Can you work these out from the model? Positions are in its coordinate system, mm. A direction names the side the tool comes from. Round coordinates to 2 decimals unless told otherwise and drop trailing zeros. Loops run counter-clockwise (first coordinate to the right, second up) from the corner with the lowest first, then second, coordinate; pieces in that order, holes last.
Autodesk Inventor part; units mm, degrees
ref_plane "YZ Plane" through (0, 0, 0) normal (1, 0, 0) x (0, 1, 0)
ref_plane "XZ Plane" through (0, 0, 0) normal (0, 1, 0) x (-1, 0, 0)
ref_plane "XY Plane" through (0, 0, 0) normal (0, 0, 1) x (1, 0, 0)
sketch "Sketch1" plane through (0, 0, 0) normal (0, 1, 0) x (-1, 0, 0)
  line L0 (0, 0) -> (-20.3922, 0)
  line L1 (-20.3922, 0) -> (-20.3922, -40.9956)
  line L2 (-20.3922, -40.9956) -> (0, -40.9956)
  line L3 (0, -40.9956) -> (0, 0)
  line L4 (1.8083, 7.7679) -> (6.8846, 7.9604)
  line L5 (-22.5838, -48.6642) -> (-27.2554, -50.6597)
  line L6 (6.8846, 7.9604) -> (-27.2554, 7.9604)
  line L7 (-27.2554, 7.9604) -> (-27.2554, -50.6597)
  line L8 (-27.2554, -50.6597) -> (6.8846, -50.6597)
  line L9 (6.8846, -50.6597) -> (6.8846, 7.9604)
  circle A0 centre (-5.0927, 3.9878) radius 1.651
  circle A1 centre (-15.2781, 3.9878) radius 1.651
  circle A2 centre (-5.0927, -44.9834) radius 1.651
  circle A3 centre (-15.2781, -44.9834) radius 1.651
  dimension "d0" = 40.9956
  dimension "d2" = 7.9756
  dimension "d3" = 5.08
  dimension "d4" = 7.9756
  dimension "d5" = 5.08
  dimension "d6" = 3.302
  dimension "d7" = 3.302
  dimension "d8" = 3.302
  dimension "d9" = 3.302
  dimension "d24" = 6.8846
  dimension "d25" = 6.8633
extrude "Extrusion1" add sketch "Sketch1" along normal blind 7.62
sketch "Sketch2" plane through (0, 0, 0) normal (0, -1, 0) x (1, 0, 0)
  line L0 (27.2554, 7.9604) -> (27.2554, -50.6597)
  line L1 (27.2554, -42.6841) -> (-6.8846, -42.6841)
  line L2 (-6.8846, -42.6841) -> (-6.8846, -50.6597)
  line L3 (-6.8846, -50.6597) -> (27.2554, -50.6597)
  line L4 (27.2554, -50.6597) -> (27.2554, -42.6841)
  point P0 (0, 0)
extrude "Extrusion2" add sketch "Sketch2" along normal blind 38.862
sketch "Sketch3" plane through (27.2554, 0, 7.9604) normal (1, 0, 0) x (0, 0, -1)
  line L0 (0, 0) -> (50.6445, -38.862)
  line L1 (50.6445, -38.862) -> (50.6445, -35.052)
  line L2 (50.6445, 0) -> (50.6445, -38.862)
  line L3 (0, 0) -> (3.81, 0)
  line L4 (0, 0) -> (50.6445, 0)
  line L5 (3.81, 0) -> (50.6445, -35.052)
  point P0 (7.9604, 0)
  dimension "d14" = 3.81
  dimension "d15" = 3.81
extrude "Extrusion3" add sketch "Sketch3" against normal blind 5.08 contours L3 L5 L1 L0
sketch "Sketch4" plane through (-6.8846, 0, -42.6841) normal (-1, 0, 0) x (0, 0, 1)
  line L0 (0, -38.862) -> (0, -35.052)
  line L1 (0, 0) -> (0, -38.862)
  line L2 (48.9049, 0) -> (45.0949, 0)
  line L3 (0, 0) -> (50.6445, 0)
  line L4 (45.0949, 0) -> (0, -35.052)
  line L5 (0, -38.862) -> (50.6445, 0)
  line L6 (50.6445, 0) -> (45.0949, 0)
  point P0 (42.6841, 0)
  dimension "d18" = 3.81
  dimension "d19" = 3.81
extrude "Extrusion4" add sketch "Sketch4" against normal blind 5.08 contours L0 L4 L2 L3 L5
sketch "Sketch5" plane through (27.2554, 7.62, -50.6597) normal (0, 0, -1) x (-1, 0, 0)
  line L0 (2.6344, -13.9998) -> (31.438, -13.9998)
  line L1 (31.438, -13.9998) -> (31.438, -42.8034)
  line L2 (31.438, -42.8034) -> (2.6344, -42.8034)
  line L3 (2.6344, -42.8034) -> (2.6344, -13.9998)
  line L4 (31.438, -13.9998) -> (2.6344, -42.8034)
  line L5 (2.6344, -13.9998) -> (31.438, -42.8034)
  line L6 (17.0362, -28.4016) -> (25.2981, -20.1398)
  line L7 (17.0362, -28.4016) -> (8.7744, -20.1398)
  line L8 (17.0362, -28.4016) -> (8.7744, -36.6634)
  line L9 (17.0362, -28.4016) -> (25.2981, -36.6634)
  line L10 (17.0362, -28.4016) -> (29.3572, -16.0807)
  line L11 (17.0362, -28.4016) -> (4.7153, -16.0807)
  line L12 (17.0362, -28.4016) -> (4.7153, -40.7225)
  line L13 (17.0362, -28.4016) -> (29.3572, -40.7225)
  circle A0 centre (25.2981, -20.1398) radius 0.508
  circle A1 centre (29.3572, -16.0807) radius 0.508
  circle A2 centre (4.7153, -16.0807) radius 0.508
  circle A3 centre (8.7744, -20.1398) radius 0.508
  circle A4 centre (8.7744, -36.6634) radius 0.508
  circle A5 centre (4.7153, -40.7225) radius 0.508
  line L14 (17.0362, -28.4016) -> (25.2981, -36.6634)
  circle A6 centre (25.2981, -36.6634) radius 0.508
  circle A7 centre (29.3572, -40.7225) radius 0.508
  circle A8 centre (17.0362, -28.4016) radius 4.1783
  point P0 (27.2554, -7.62)
  dimension "d22" = 28.8036
  dimension "d26" = 28.8036
  dimension "d27" = 11.684
  dimension "d28" = 11.684
  dimension "d29" = 11.684
  dimension "d30" = 17.4244
  dimension "d31" = 17.4244
  dimension "d32" = 17.4244
  dimension "d33" = 17.4244
  dimension "d34" = 1.016
  dimension "d35" = 1.016
  dimension "d36" = 1.016
  dimension "d37" = 1.016
  dimension "d38" = 1.016
  dimension "d39" = 1.016
  dimension "d40" = 11.684
  dimension "d41" = 1.016
  dimension "d42" = 1.016
  dimension "d43" = 8.3566
extrude "Extrusion5" cut sketch "Sketch5" against normal blind 9.906 contours A2 L5 | L5 A2 | A1 L4 | L4 A1 | A5 L4 | L4 A5 | A7 L5 | L5 A7 | A3 L5 | L5 A3 | A0 L4 | L4 A0 | A4 L4 | L4 A4 | A6 L5 | L5 A6 | A8 L4 L5 | L5 L4 A8 | A8 L5 L4 | L4 L5 A8
(1) If we mould it in two halves opening along X, with no side actions, what happens to faces 1 (the flat face through (0, 4, -21)), 2 (the flat face through (27.255, 0.2, -27.5)), 3 (the flat face through (10, 4, 7.96)), 4 (the flat face through (-6.885, 0.2, -28.3))? For each: released by +X, released by -X, zero draft, split by the parting line, or undercut.
Worked answers:
face 1: undercut
face 2: released by +X
face 3: zero draft
face 4: released by -X
(2) If we section it at B-B, the plane z = -9: List the corners of the cut face in (x, y) for me, then the cut area to 3 significant figures.
Worked answers:
outline: (-6.88, -13.01) - (-1.8, -13.01) - (-1.8, -8.87) - (-6.88, -8.87) - close; (-6.88, 0) - (0, 0) - (0, 7.62) - (-6.88, 7.62) - close; (20.39, 0) - (27.26, 0) - (27.26, 7.62) - (20.39, 7.62) - close; (22.18, -13.01) - (27.26, -13.01) - (27.26, -9.84) - (22.18, -9.84) - close
area: 142 mm2
(3) Will these pins go through, and if not, where does the flat tip stop? P1, Ø11.5, axis at y = -27, z = -15, coming from the -X side; P2, Ø1.2, axis at x = 1.96, y = -29.04, coming from the +Z side; P3, Ø6, axis at y = -0.5, z = -10, coming from the -X side; P4, Ø1.2, axis at x = 22.54, y = -33.1, coming from the +Z side.
Worked answers:
P1: passes through
P2: stops at z = -42.68
P3: stops at x = -6.88
P4: stops at z = -34.39
(4) If we section it at C-C, the plane x = 9: List the corners of the cut face in (y, z) for me.
Worked answers:
outline: (-38.86, -50.66) - (-24.78, -50.66) - (-24.78, -42.68) - (-38.86, -42.68) - close; (-16.79, -50.66) - (7.62, -50.66) - (7.62, -41) - (0, -41) - (0, -42.68) - (-16.79, -42.68) - close; (0, 0) - (7.62, 0) - (7.62, 7.96) - (0, 7.96) - close
(5) If I drill on line 1 (X direction, y = -1, z = 4); line 2 (X direction, y = 2, z = -17); line 3 (Z direction, x = 0.5, y = -1), over which ranges is the centre line in solid material (lowest first)?
Worked answers:
line 1: x = -6.88 to -1.8, 22.18 to 27.26
line 2: x = -6.88 to 0, 20.39 to 27.26
line 3: z = -50.66 to -42.68
(6) If we section it at D-D, the plane y = -31: List the corners of the cut face in (x, z) for me, then the cut area to 3 significant figures.
Worked answers:
outline: (-6.88, -50.66) - (27.26, -50.66) - (27.26, -42.68) - (-6.88, -42.68) - close; (-6.88, -37.47) - (-1.8, -37.47) - (-1.8, -32.44) - (-6.88, -32.44) - close; (22.18, -37.27) - (27.26, -37.27) - (27.26, -32.44) - (22.18, -32.44) - close
area: 322 mm2
(7) If we section it at A-A, the plane y = -21.5: List the corners of the cut face in (x, z) for me.
Worked answers:
outline: (-6.88, -50.66) - (6.1, -50.66) - (6.1, -42.68) - (-6.88, -42.68) - close; (-6.88, -25.25) - (-1.8, -25.25) - (-1.8, -20.06) - (-6.88, -20.06) - close; (14.34, -50.66) - (27.26, -50.66) - (27.26, -42.68) - (14.34, -42.68) - close; (22.18, -24.58) - (27.26, -24.58) - (27.26, -20.06) - (22.18, -20.06) - close
(8) For faces 5 (the flat face through (20.392, 4, -20)), 6 (the flat face through (-1, 7.62, -21)), 7 (the flat face through (-1.805, -19.3, -17.5)), 8 (the flat face through (-1, 0, -17)), 9 (the cylindrical face through (6.31, 3.76, -46.1)), which set-ups out of +Z, -Z, +X, -X, +Y, -Y let a thin tool reach every point of the face, with its end or its side?
Worked answers:
face 5: +Y, -Y
face 6: +Z, -Z, +X, -X, +Y
face 7: +Z, -Y
face 8: none
face 9: +Y
